Could you check a few things on this drawing? It's one solid part, dimensions in mm from its lowest x, y, z. A direction names the side the tool comes from. Round coordinates to 2 decimals unless told otherwise and drop trailing zeros. Write each loop counter-clockwise with the first axis right and the second up, starting at its lowest first coordinate (ties: lowest second). Pieces come first, ordered by that corner, then holes. Notation, with made-up numbers: M 22,81 L 79,81 A11 cw 79,87 Z; hole C 30,-35.5 d4. An arc over 180 degrees is marked long. One line per question, with ' | ' between items. Start each with the question number.
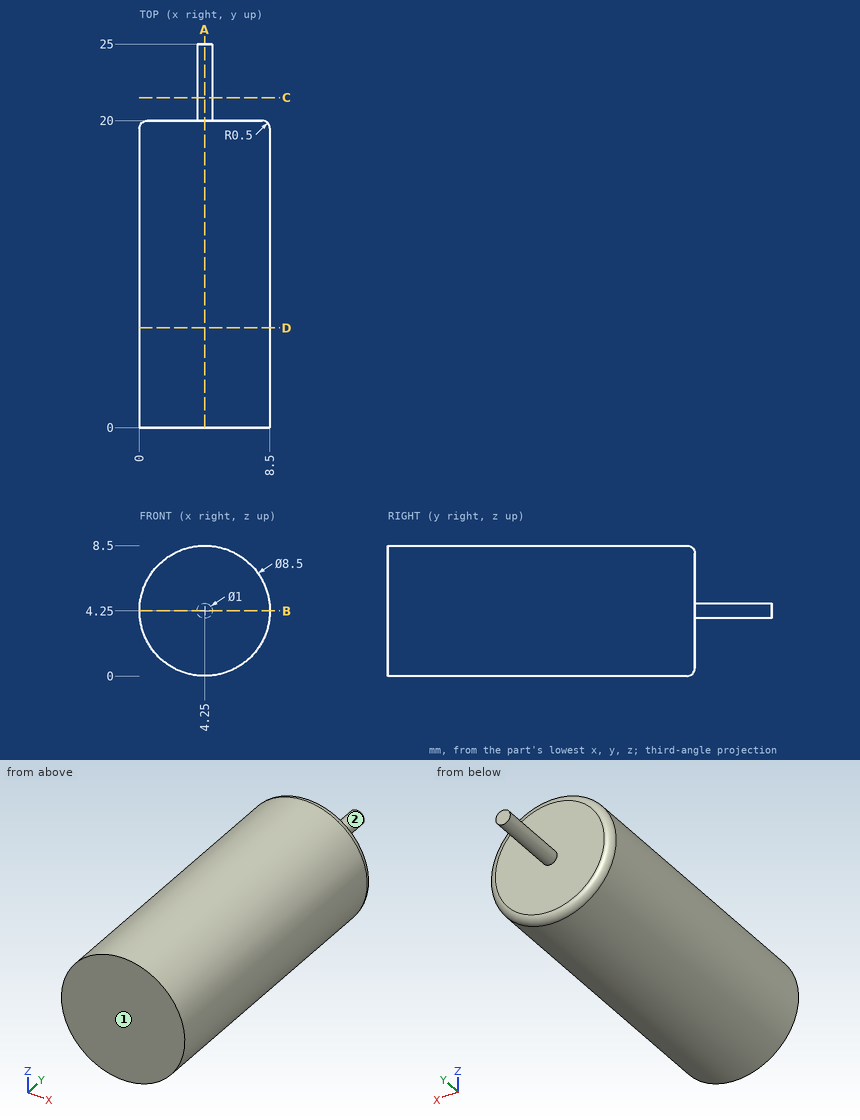
1. I need wall thicknesses on line 1 along Y through (x, z) = (4.25, 7); line 2 along X through (y, z) = (6.25, 6.25). Which ranges of each line are inside material? Lowest first, please. Write a range as from..to.
2. Suppose I cut it at B-B (z = 4.25). Write out the boundary of the cut face in (x, y), and give its area (3 significant figures).
3. I'm going to push flat-ended pins straight in: P1, Ø1, axis at y = 14, z = 6, coming from the -X side; P2, Ø5, axis at x = 1.5, z = 2.5, coming from the +Y side. Where does each tip first touch, or does it pass through?
4. Suppose I cut it at C-C (y = 21.5). Write out the boundary of the cut face in (x, z), and give its area (3 significant figures).
5. Suppose I cut it at D-D (y = 6.5). Write out the boundary of the cut face in (x, z).
6. Which directions (+Z, -Z, +X, -X, +Y, -Y) give clear straight access to the entire face, cutting with the end or side of a thin tool? Please do the marked faces 1 and 2.
7. Suppose I cut it at A-A (x = 4.25). Write out the boundary of the cut face in (y, z), and give its area (3 significant figures).
Computed:
1) line 1: y = 0..20 | line 2: x = 0.5..8
2) outline: M 0,0 L 8.5,0 L 8.5,19.5 A0.5 ccw 8,20 L 4.75,20 L 4.75,25 L 3.75,25 L 3.75,20 L 0.5,20 A0.5 ccw 0,19.5 Z | area: 175 mm²
3) P1: stops at x = 0.19 | P2: stops at y = 20
4) outline: C 4.25,4.25 d1 | area: 0.785 mm²
5) outline: C 4.25,4.25 d8.5
6) face 1: +Z, -Z, +X, -X, -Y | face 2: +Y
7) outline: M 0,0 L 19.5,0 A0.5 ccw 20,0.5 L 20,3.75 L 25,3.75 L 25,4.75 L 20,4.75 L 20,8 A0.5 ccw 19.5,8.5 L 0,8.5 Z | area: 175 mm²
